Can you work these out from the model? Positions are in its coordinate system, mm. A direction names the side the tool comes from. Round coordinates to 2 decimals unless told otherwise and drop trailing zeros. Loops run counter-clockwise (first coordinate to the right, second up) from the corner with the lowest first, then second, coordinate; pieces in that order, holes last.
(1) I want a section at B-B on x = 60. Write out the boundary of the cut face in (y, z), plus the area to 3 significant figures.
(2) Thinking about a two-plate mould opening in Y: for faces 3 (the face through (10, 2, 7)), 4 (the face through (2.85, 63.99, 1.97)), 5 (the face through (38.526, 8.352, 0.986)), which applies, released by +Y, released by -Y, zero draft, split by the parting line, or undercut?
(3) I want a section at D-D on z = 7. Write out the boundary of the cut face in (x, y).
(4) Will these pins go through, and if not, where does the flat tip stop? pin 1 Ø4.5 at (x, y) = (20, 47) entering from -Z; pin 2 Ø6 at (x, y) = (51.5, 27) entering from +Z; pin 3 Ø1.5 at (y, z) = (1.5, 6) entering from -X.
(5) I want a section at A-A on y = 37. Give the number of separate pieces and of enclosed holes in the cut face, plus the area to 3 significant figures.
(6) Which directions (+Z, -Z, +X, -X, +Y, -Y) give clear straight access to the entire face, cutting with the end or side of a thin tool? Please do faces 1 (the face through (76, 10, 7)), 2 (the face through (40, 45, 1)).
(7) I want a section at C-C on z = 3. Write out the boundary of the cut face in (x, y).
(8) If I drill on line 1 along Z through (x, y) = (34.5, 54); line 2 along Y through (x, z) = (5, 10.25); line 3 along Y through (x, z) = (5.5, 3), over which ranges is the centre line in solid material (lowest first)?
from build123d import *

# Parameters (mm, degrees)
ESQUISSE1_R             = 2
BOSS_EXTRU_1_DEPTH      = 2
BOSS_EXTRU_2_DEPTH      = 10
CHANFREIN1_SIZE         = 8
CHANFREIN1_SIZE2        = 1.410615846
CHANFREIN1_PART_2_SIZE  = 8
CHANFREIN1_PART_2_SIZE2 = 1.410615846
CHANFREIN1_PART_3_SIZE  = 8
CHANFREIN1_PART_3_SIZE2 = 1.410615846
CHANFREIN1_PART_4_SIZE  = 8
CHANFREIN1_PART_4_SIZE2 = 1.410615846


with BuildPart() as part:
    # Esquisse1 → Boss.-Extru.1 (new body)
    with BuildSketch(Plane.XY):
        with BuildLine():
            Line((10, 0), (68, 0))
            ThreePointArc((68, 0), (75.071067812, 2.928932188), (78, 10))
            Line((78, 10), (78, 57))
            ThreePointArc((78, 57), (75.071067812, 64.071067812), (68, 67))
            Line((68, 67), (10, 67))
            ThreePointArc((10, 67), (2.928932188, 64.071067812), (0, 57))
            Line((0, 57), (0, 10))
            ThreePointArc((0, 10), (2.928932188, 2.928932188), (10, 0))
        make_face()
        with Locations((10, 57)):
            Circle(ESQUISSE1_R, mode=Mode.SUBTRACT)
        with Locations((20, 57)):
            Circle(ESQUISSE1_R, mode=Mode.SUBTRACT)
        with Locations((30, 57)):
            Circle(ESQUISSE1_R, mode=Mode.SUBTRACT)
        with Locations((40, 57)):
            Circle(ESQUISSE1_R, mode=Mode.SUBTRACT)
        with Locations((50, 57)):
            Circle(ESQUISSE1_R, mode=Mode.SUBTRACT)
        with Locations((60, 57)):
            Circle(ESQUISSE1_R, mode=Mode.SUBTRACT)
        with Locations((70, 57)):
            Circle(ESQUISSE1_R, mode=Mode.SUBTRACT)
        with Locations((20, 47)):
            Circle(ESQUISSE1_R, mode=Mode.SUBTRACT)
        with Locations((30, 47)):
            Circle(ESQUISSE1_R, mode=Mode.SUBTRACT)
        with Locations((40, 47)):
            Circle(ESQUISSE1_R, mode=Mode.SUBTRACT)
        with Locations((50, 47)):
            Circle(ESQUISSE1_R, mode=Mode.SUBTRACT)
        with Locations((60, 47)):
            Circle(ESQUISSE1_R, mode=Mode.SUBTRACT)
        with Locations((70, 47)):
            Circle(ESQUISSE1_R, mode=Mode.SUBTRACT)
        with Locations((20, 37)):
            Circle(ESQUISSE1_R, mode=Mode.SUBTRACT)
        with Locations((30, 37)):
            Circle(ESQUISSE1_R, mode=Mode.SUBTRACT)
        with Locations((40, 37)):
            Circle(ESQUISSE1_R, mode=Mode.SUBTRACT)
        with Locations((50, 37)):
            Circle(ESQUISSE1_R, mode=Mode.SUBTRACT)
        with Locations((60, 37)):
            Circle(ESQUISSE1_R, mode=Mode.SUBTRACT)
        with Locations((70, 37)):
            Circle(ESQUISSE1_R, mode=Mode.SUBTRACT)
        with Locations((20, 27)):
            Circle(ESQUISSE1_R, mode=Mode.SUBTRACT)
        with Locations((30, 27)):
            Circle(ESQUISSE1_R, mode=Mode.SUBTRACT)
        with Locations((40, 27)):
            Circle(ESQUISSE1_R, mode=Mode.SUBTRACT)
        with Locations((50, 27)):
            Circle(ESQUISSE1_R, mode=Mode.SUBTRACT)
        with Locations((60, 27)):
            Circle(ESQUISSE1_R, mode=Mode.SUBTRACT)
        with Locations((70, 27)):
            Circle(ESQUISSE1_R, mode=Mode.SUBTRACT)
        with Locations((20, 17)):
            Circle(ESQUISSE1_R, mode=Mode.SUBTRACT)
        with Locations((30, 17)):
            Circle(ESQUISSE1_R, mode=Mode.SUBTRACT)
        with Locations((40, 17)):
            Circle(ESQUISSE1_R, mode=Mode.SUBTRACT)
        with Locations((50, 17)):
            Circle(ESQUISSE1_R, mode=Mode.SUBTRACT)
        with Locations((60, 17)):
            Circle(ESQUISSE1_R, mode=Mode.SUBTRACT)
        with Locations((70, 17)):
            Circle(ESQUISSE1_R, mode=Mode.SUBTRACT)
        with Locations((20, 7)):
            Circle(ESQUISSE1_R, mode=Mode.SUBTRACT)
        with Locations((30, 7)):
            Circle(ESQUISSE1_R, mode=Mode.SUBTRACT)
        with Locations((40, 7)):
            Circle(ESQUISSE1_R, mode=Mode.SUBTRACT)
        with Locations((50, 7)):
            Circle(ESQUISSE1_R, mode=Mode.SUBTRACT)
        with Locations((60, 7)):
            Circle(ESQUISSE1_R, mode=Mode.SUBTRACT)
        with Locations((70, 7)):
            Circle(ESQUISSE1_R, mode=Mode.SUBTRACT)
        with Locations((10, 47)):
            Circle(ESQUISSE1_R, mode=Mode.SUBTRACT)
        with Locations((10, 37)):
            Circle(ESQUISSE1_R, mode=Mode.SUBTRACT)
        with Locations((10, 27)):
            Circle(ESQUISSE1_R, mode=Mode.SUBTRACT)
        with Locations((10, 17)):
            Circle(ESQUISSE1_R, mode=Mode.SUBTRACT)
        with Locations((10, 7)):
            Circle(ESQUISSE1_R, mode=Mode.SUBTRACT)
    extrude(amount=BOSS_EXTRU_1_DEPTH)

    # Esquisse2 → Boss.-Extru.2 (add)
    with BuildSketch(Plane.XY.offset(2)):
        with BuildLine():
            Line((10, 67), (10, 64))
            ThreePointArc((10, 64), (5.050252532, 61.949747468), (3, 57))
            Line((3, 57), (0, 57))
            ThreePointArc((0, 57), (2.928932188, 64.071067812), (10, 67))
        make_face()
        with BuildLine():
            Line((0, 10), (3, 10))
            ThreePointArc((3, 10), (5.050252532, 5.050252532), (10, 3))
            Line((10, 3), (10, 0))
            ThreePointArc((10, 0), (2.928932188, 2.928932188), (0, 10))
        make_face()
        with BuildLine():
            Line((75, 10), (78, 10))
            ThreePointArc((78, 10), (75.071067812, 2.928932188), (68, 0))
            Line((68, 0), (68, 3))
            ThreePointArc((68, 3), (72.949747468, 5.050252532), (75, 10))
        make_face()
        with BuildLine():
            Line((78, 57), (75, 57))
            ThreePointArc((75, 57), (72.949747468, 61.949747468), (68, 64))
            Line((68, 64), (68, 67))
            ThreePointArc((68, 67), (75.071067812, 64.071067812), (78, 57))
        make_face()
    extrude(amount=BOSS_EXTRU_2_DEPTH)

    # Chanfrein1
    chanfrein1_edges = [part.edges().sort_by_distance(p)[0] for p in [
        (2.928932188, 64.071067812, 12),
    ]]
    chanfrein1_side = [part.faces().sort_by_distance(p)[0] for p in [
        (2.928932188, 64.071067812, 6),
    ]]
    chamfer(chanfrein1_edges, length=CHANFREIN1_SIZE, length2=CHANFREIN1_SIZE2, reference=chanfrein1_side[0])

    # Chanfrein1 part 2
    chanfrein1_part_2_edges = [part.edges().sort_by_distance(p)[0] for p in [
        (2.928932188, 2.928932188, 12),
    ]]
    chanfrein1_part_2_side = [part.faces().sort_by_distance(p)[0] for p in [
        (2.928932188, 2.928932188, 6),
    ]]
    chamfer(chanfrein1_part_2_edges, length=CHANFREIN1_PART_2_SIZE, length2=CHANFREIN1_PART_2_SIZE2, reference=chanfrein1_part_2_side[0])

    # Chanfrein1 part 3
    chanfrein1_part_3_edges = [part.edges().sort_by_distance(p)[0] for p in [
        (75.071067812, 64.071067812, 12),
    ]]
    chanfrein1_part_3_side = [part.faces().sort_by_distance(p)[0] for p in [
        (75.071067812, 64.071067812, 6),
    ]]
    chamfer(chanfrein1_part_3_edges, length=CHANFREIN1_PART_3_SIZE, length2=CHANFREIN1_PART_3_SIZE2, reference=chanfrein1_part_3_side[0])

    # Chanfrein1 part 4
    chanfrein1_part_4_edges = [part.edges().sort_by_distance(p)[0] for p in [
        (75.071067812, 2.928932188, 12),
    ]]
    chanfrein1_part_4_side = [part.faces().sort_by_distance(p)[0] for p in [
        (75.071067812, 2.928932188, 6),
    ]]
    chamfer(chanfrein1_part_4_edges, length=CHANFREIN1_PART_4_SIZE, length2=CHANFREIN1_PART_4_SIZE2, reference=chanfrein1_part_4_side[0])


solid = part.part
Filled sheet:
1. outline: (0, 0) - (5, 0) - (5, 2) - (0, 2) - close; (9, 0) - (15, 0) - (15, 2) - (9, 2) - close; (19, 0) - (25, 0) - (25, 2) - (19, 2) - close; (29, 0) - (35, 0) - (35, 2) - (29, 2) - close; (39, 0) - (45, 0) - (45, 2) - (39, 2) - close; (49, 0) - (55, 0) - (55, 2) - (49, 2) - close; (59, 0) - (67, 0) - (67, 2) - (59, 2) - close
1. area: 86.0 mm2
2. face 3: zero draft
2. face 4: released by +Y
2. face 5: undercut
3. outline: (0.53, 10) arc R9.47 ccw to (10, 0.53) - (10, 3) arc R7 cw to (3, 10) - close; (0.53, 57) - (3, 57) arc R7 cw to (10, 64) - (10, 66.47) arc R9.47 ccw to start; (68, 0.53) arc R9.47 ccw to (77.47, 10) - (75, 10) arc R7 cw to (68, 3) - close; (68, 64) arc R7 cw to (75, 57) - (77.47, 57) arc R9.47 ccw to (68, 66.47) - close
4. pin 1: stops at z = 0
4. pin 2: stops at z = 2
4. pin 3: stops at x = 4.23
5. separate pieces: 8
5. enclosed holes: 0
5. area: 100 mm2
6. face 1: +Z, +X, -X
6. face 2: +Z, -Z
7. outline: (0, 10) arc R10 ccw to (10, 0) - (10, 3) arc R7 cw to (3, 10) - close; (0, 57) - (3, 57) arc R7 cw to (10, 64) - (10, 67) arc R10 ccw to start; (68, 0) arc R10 ccw to (78, 10) - (75, 10) arc R7 cw to (68, 3) - close; (68, 64) arc R7 cw to (75, 57) - (78, 57) arc R10 ccw to (68, 67) - close
8. line 1: z = 0 to 2
8. line 2: y = 2.64 to 5.1, 61.9 to 64.36
8. line 3: y = 1.07 to 4.64, 62.36 to 65.93
